For this review, take the finished solid that the model builds, in its own axes (mm). A direction names the side the tool comes from. Give positions to 0.01 mm unless a question says otherwise; leave off trailing zeros. Loops run counter-clockwise (first coordinate to the right, second up) from the corner with the lowest first, then second, coordinate; pieces in that order, holes last. Notation, with made-up numbers: (14.5, -0.5) -> (34.5, -0.5) arc R11 ccw to (34.5, 18.5) -> close; hole circle Ø3 at (88, 36.25). An arc over 180 degrees is marked (long way). Write each question's results on one line, items separated by ' | '. Start each with the question number.
```python
from build123d import *

# Parameters (mm, degrees)
SKETCH1_W                     = 190.5
SKETCH1_H                     = 101.6
BOSS_EXTRUDE1_DEPTH           = 1.5875
CONVERT_SOLID1_START          = -95.25
CONVERT_SOLID1_OUTLINE_W      = 3.175
CONVERT_SOLID1_OUTLINE_H      = 101.6
CONVERT_SOLID1_DEPTH          = 190.5
SKETCH30_R                    = 12.770921212
CUT_EXTRUDE6_DEPTH            = 38.1
SKETCH35_W                    = 139.601875342
SKETCH35_H                    = 6.35
CUT_EXTRUDE7_DEPTH            = 0.254
EDGE_FLANGE1_STRIP_W          = 39.05
EDGE_FLANGE1_STRIP_H          = 4.7625
EDGE_FLANGE1_STRIP_CUT_DEPTH  = 25.449062329
EDGE_FLANGE1_RELIEF_W         = 41.43125
EDGE_FLANGE1_RELIEF_H         = 2.38125
EDGE_FLANGE1_RELIEF_CUT_DEPTH = 4.7625
EDGE_FLANGE1_DEPTH            = 25.449062329
EDGE_FLANGE2_STRIP_W          = 39.05
EDGE_FLANGE2_STRIP_H          = 4.7625
EDGE_FLANGE2_STRIP_CUT_DEPTH  = 25.449062329
EDGE_FLANGE2_RELIEF_W         = 41.43125
EDGE_FLANGE2_RELIEF_H         = 2.38125
EDGE_FLANGE2_RELIEF_CUT_DEPTH = 4.7625
EDGE_FLANGE2_DEPTH            = 25.449062329
SKETCH45_W                    = 4.7625
SKETCH45_H                    = 0.000254
CUT_EXTRUDE10_DEPTH           = 25.4
EDGE_FLANGE4_STRIP_W          = 39.05
EDGE_FLANGE4_STRIP_H          = 4.7625
EDGE_FLANGE4_STRIP_CUT_DEPTH  = 25.4
EDGE_FLANGE4_RELIEF_W         = 41.43125
EDGE_FLANGE4_RELIEF_H         = 2.38125
EDGE_FLANGE4_RELIEF_CUT_DEPTH = 4.7625
EDGE_FLANGE4_DEPTH            = 25.4
FILLET9_R                     = 25.4
CUT_EXTRUDE11_DEPTH           = 25.4
FILLET10_R                    = 25.4
SKETCH53_R                    = 2.54
CUT_EXTRUDE12_DEPTH           = 4.7625
SKETCH54_R                    = 2.54
CUT_EXTRUDE13_DEPTH           = 4.7625
SKETCH55_R                    = 9.525
SKETCH55_R_2                  = 2.54
CUT_EXTRUDE14_DEPTH           = 4.7625


# Read off the part's stored shape, not the designer's step: Convert-Solid1
# Sheet-metal steps are written as plain solids
with BuildPart() as part:
    # Sketch1 → Boss-Extrude1 (new body)
    with BuildSketch(Plane(origin=(0, 0, 0), x_dir=(1, 0, 0), z_dir=(0, 1, 0))):
        Rectangle(SKETCH1_W, SKETCH1_H)
    extrude(amount=BOSS_EXTRUDE1_DEPTH)

    # Convert-Solid1 outline → Convert-Solid1 (add)
    with BuildSketch(Plane.YZ.offset(CONVERT_SOLID1_START)):
        with Locations((-1.5875, 0)):
            Rectangle(CONVERT_SOLID1_OUTLINE_W, CONVERT_SOLID1_OUTLINE_H)
    extrude(amount=CONVERT_SOLID1_DEPTH)

    # Sketch30 → Cut-Extrude6 (cut)
    with BuildSketch(Plane(origin=(0, -3.175, 0), x_dir=(-1, 0, 0), z_dir=(0, -1, 0))):
        with Locations(Location((0, -25.504506424, 0), (0, 0, 90))):
            Circle(SKETCH30_R)
    extrude(amount=-CUT_EXTRUDE6_DEPTH, mode=Mode.SUBTRACT)

    # Sketch35 → Cut-Extrude7 (cut)
    with BuildSketch(Plane(origin=(0, 0, -50.8), x_dir=(-1, 0, 0), z_dir=(0, 0, -1))):
        Rectangle(SKETCH35_W, SKETCH35_H)
    extrude(amount=-CUT_EXTRUDE7_DEPTH, mode=Mode.SUBTRACT)

    # Edge-Flange1 strip (across the edge) → Edge-Flange1 strip cut (cut)
    with BuildSketch(Plane(origin=(95.25, 1.5875, -50.8), x_dir=(0, 0, 1), z_dir=(-1, 0, 0))):
        with Locations((-4.7625, -2.38125)):
            Rectangle(EDGE_FLANGE1_STRIP_W, EDGE_FLANGE1_STRIP_H)
    extrude(amount=EDGE_FLANGE1_STRIP_CUT_DEPTH, mode=Mode.SUBTRACT)

    # Edge-Flange1 relief (on the sheet) → Edge-Flange1 relief cut (cut)
    with BuildSketch(Plane(origin=(95.25, 1.5875, -36.0375), x_dir=(0, 0, 1), z_dir=(0, 1, 0))):
        with Locations((-18.334375, -26.639687329)):
            Rectangle(EDGE_FLANGE1_RELIEF_W, EDGE_FLANGE1_RELIEF_H)
    extrude(amount=-EDGE_FLANGE1_RELIEF_CUT_DEPTH, mode=Mode.SUBTRACT)

    # Edge-Flange1 section (across the edge) → Edge-Flange1 (add)
    with BuildSketch(Plane(origin=(95.25, 1.5875, -50.8), x_dir=(0, 0, 1), z_dir=(-1, 0, 0))):
        with BuildLine():
            Line((0, 10), (0, 46.0375))
            Line((0, 46.0375), (4.7625, 46.0375))
            Line((4.7625, 46.0375), (4.7625, 10))
            ThreePointArc((4.7625, 10), (7.691432188, 2.928932188), (14.7625, 0))
            Line((14.7625, 0), (14.7625, -4.7625))
            ThreePointArc((14.7625, -4.7625), (4.323836143, -0.438663857), (0, 10))
        make_face()
    extrude(amount=EDGE_FLANGE1_DEPTH)

    # Edge-Flange2 strip (across the edge) → Edge-Flange2 strip cut (cut)
    with BuildSketch(Plane(origin=(-69.800937671, 1.5875, -50.8), x_dir=(0, 0, 1), z_dir=(-1, 0, 0))):
        with Locations((-4.7625, -2.38125)):
            Rectangle(EDGE_FLANGE2_STRIP_W, EDGE_FLANGE2_STRIP_H)
    extrude(amount=EDGE_FLANGE2_STRIP_CUT_DEPTH, mode=Mode.SUBTRACT)

    # Edge-Flange2 relief (on the sheet) → Edge-Flange2 relief cut (cut)
    with BuildSketch(Plane(origin=(-69.800937671, 1.5875, -36.0375), x_dir=(0, 0, 1), z_dir=(0, 1, 0))):
        with Locations((-18.334375, 1.190625)):
            Rectangle(EDGE_FLANGE2_RELIEF_W, EDGE_FLANGE2_RELIEF_H)
    extrude(amount=-EDGE_FLANGE2_RELIEF_CUT_DEPTH, mode=Mode.SUBTRACT)

    # Edge-Flange2 section (across the edge) → Edge-Flange2 (add)
    with BuildSketch(Plane(origin=(-69.800937671, 1.5875, -50.8), x_dir=(0, 0, 1), z_dir=(-1, 0, 0))):
        with BuildLine():
            Line((0, 10), (0, 46.0375))
            Line((0, 46.0375), (4.7625, 46.0375))
            Line((4.7625, 46.0375), (4.7625, 10))
            ThreePointArc((4.7625, 10), (7.691432188, 2.928932188), (14.7625, 0))
            Line((14.7625, 0), (14.7625, -4.7625))
            ThreePointArc((14.7625, -4.7625), (4.323836143, -0.438663857), (0, 10))
        make_face()
    extrude(amount=EDGE_FLANGE2_DEPTH)

    # Sketch45 → Cut-Extrude10 (cut)
    with BuildSketch(Plane(origin=(0, 1.5875, 0), x_dir=(1, 0, 0), z_dir=(0, 1, 0))):
        with Locations((-92.86875, -25.399873)):
            Rectangle(SKETCH45_W, SKETCH45_H)
        with Locations((-92.86875, 0.000381)):
            Rectangle(SKETCH45_W, SKETCH45_H)
    extrude(amount=-CUT_EXTRUDE10_DEPTH, mode=Mode.SUBTRACT)

    # Edge-Flange4 strip (across the edge) → Edge-Flange4 strip cut (cut)
    with BuildSketch(Plane(origin=(-95.25, 1.5875, -0.000254), x_dir=(1, 0, 0), z_dir=(0, 0, 1))):
        with Locations((-4.7625, -2.38125)):
            Rectangle(EDGE_FLANGE4_STRIP_W, EDGE_FLANGE4_STRIP_H)
    extrude(amount=EDGE_FLANGE4_STRIP_CUT_DEPTH, mode=Mode.SUBTRACT)

    # Edge-Flange4 relief (on the sheet) → Edge-Flange4 relief cut (cut)
    with BuildSketch(Plane(origin=(-80.4875, 1.5875, -0.000254), x_dir=(1, 0, 0), z_dir=(0, 1, 0))):
        with Locations((-18.334375, 1.190625)):
            Rectangle(EDGE_FLANGE4_RELIEF_W, EDGE_FLANGE4_RELIEF_H)
        with Locations((-18.334375, -26.590625)):
            Rectangle(EDGE_FLANGE4_RELIEF_W, EDGE_FLANGE4_RELIEF_H)
    extrude(amount=-EDGE_FLANGE4_RELIEF_CUT_DEPTH, mode=Mode.SUBTRACT)

    # Edge-Flange4 section (across the edge) → Edge-Flange4 (add)
    with BuildSketch(Plane(origin=(-95.25, 1.5875, -0.000254), x_dir=(1, 0, 0), z_dir=(0, 0, 1))):
        with BuildLine():
            Line((0, 10), (0, 20.6375))
            Line((0, 20.6375), (4.7625, 20.6375))
            Line((4.7625, 20.6375), (4.7625, 10))
            ThreePointArc((4.7625, 10), (7.691432188, 2.928932188), (14.7625, 0))
            Line((14.7625, 0), (14.7625, -4.7625))
            ThreePointArc((14.7625, -4.7625), (4.323836143, -0.438663857), (0, 10))
        make_face()
    extrude(amount=EDGE_FLANGE4_DEPTH)

    # Fillet9
    # the kernel refuses this fillet: 25.4 mm, written as the material it takes off along each edge
    with BuildSketch(Plane(origin=(-67.419687671, 61.417239936, -50.546), x_dir=(1, 0, 0), z_dir=(0, -1, 0))) as fillet9_piece_1:
        with BuildLine():
            CenterArc((23.931895975, 25.4), FILLET9_R, 199.575530564, 70.424469436)
            Line((0, 16.88975), (-0.478637919, 16.719545))
            ThreePointArc((-0.478637919, 16.719545), (-0.508, 8.444875), (-0.508, 0))
            Line((-0.508, 0), (0, -0.508))
            Line((0, -0.508), (23.931895975, -0.508))
            Line((23.931895975, -0.508), (23.931895975, 0))
        make_face()
    extrude(amount=124.421979873, mode=Mode.SUBTRACT)
    with BuildSketch(Plane(origin=(67.419687671, 61.417239936, -50.546), x_dir=(0, 0, 1), z_dir=(0, -1, 0))) as fillet9_piece_2:
        with BuildLine():
            CenterArc((25.4, 23.931895975), FILLET9_R, 180, 70.424469436)
            Line((0, 23.931895975), (-0.508, 23.931895975))
            Line((-0.508, 23.931895975), (-0.508, 0))
            Line((-0.508, 0), (0, -0.508))
            ThreePointArc((0, -0.508), (8.444875, -0.508), (16.719545, -0.478637919))
            Line((16.719545, -0.478637919), (16.88975, 0))
        make_face()
    extrude(amount=124.421979873, mode=Mode.SUBTRACT)

    # Sketch52 → Cut-Extrude11 (cut)
    with BuildSketch(Plane.XZ.offset(3.175)):
        with BuildLine():
            ThreePointArc((62.156767956, 50.8), (84.936935051, 40.486935051), (95.25, 17.706767956))
            Line((95.25, 17.706767956), (95.25, 50.8))
            Line((95.25, 50.8), (62.156767956, 50.8))
        make_face()
    extrude(amount=-CUT_EXTRUDE11_DEPTH, mode=Mode.SUBTRACT)

    # Fillet10
    # the kernel refuses this fillet: 25.4 mm, written as the material it takes off along each edge
    with BuildSketch(Plane(origin=(-95.25, 64.807891195, 50.8), x_dir=(1, 0, 0), z_dir=(0, -1, 0))) as fillet10_piece_1:
        with BuildLine():
            CenterArc((25.288156478, -25.4), FILLET10_R, 90, 84.621196501)
            Line((0, -23.019004), (-0.50576313, -22.97138408))
            ThreePointArc((-0.50576313, -22.97138408), (-0.508, -11.509502), (-0.508, 0))
            Line((-0.508, 0), (0, 0.508))
            Line((0, 0.508), (25.288156478, 0.508))
            Line((25.288156478, 0.508), (25.288156478, 0))
        make_face()
    extrude(amount=131.203282389, mode=Mode.SUBTRACT)

    # Sketch53 → Cut-Extrude12 (cut)
    with BuildSketch(Plane.ZY.offset(95.25)):
        with Locations(Location((6.349746, 17.9375, 0), (0, 0, 270))):
            Circle(SKETCH53_R)
        with Locations(Location((19.049746, 17.9375, 0), (0, 0, 270))):
            Circle(SKETCH53_R)
    extrude(amount=-CUT_EXTRUDE12_DEPTH, mode=Mode.SUBTRACT)

    # Sketch54 → Cut-Extrude13 (cut)
    with BuildSketch(Plane(origin=(0, 0, -50.8), x_dir=(-1, 0, 0), z_dir=(0, 0, -1))):
        with Locations(Location((-82.55, 34.925, 0), (0, 0, 90))):
            Circle(SKETCH54_R)
        with Locations(Location((82.55, 34.925, 0), (0, 0, 90))):
            Circle(SKETCH54_R)
    extrude(amount=-CUT_EXTRUDE13_DEPTH, mode=Mode.SUBTRACT)

    # Sketch55 → Cut-Extrude14 (cut)
    with BuildSketch(Plane.XZ.offset(3.175)):
        with Locations(Location((-39.37, -22.688605117, 0), (0, 0, 270))):
            Circle(SKETCH55_R)
        with Locations(Location((39.37, -22.688605117, 0), (0, 0, 270))):
            Circle(SKETCH55_R)
        with Locations(Location((-17.001810213, -34.722893033, 0), (0, 0, 270))):
            Circle(SKETCH55_R_2)
        with Locations(Location((-61.002047674, -9.376410953, 0), (0, 0, 270))):
            Circle(SKETCH55_R_2)
        with Locations(Location((61.002047674, -9.376410953, 0), (0, 0, 270))):
            Circle(SKETCH55_R_2)
        with Locations(Location((17.001810213, -34.722893033, 0), (0, 0, 270))):
            Circle(SKETCH55_R_2)
    extrude(amount=-CUT_EXTRUDE14_DEPTH, mode=Mode.SUBTRACT)


solid = part.part
```
1. We need section D-D (y = 5). Write out the cut boundary in (x, z), plus the area to 3 significant figures.
2. Wall thickness on L1, parallel to Z at x = -39, y = -1; L2, parallel to Y at x = 27, z = 32 (1 decimal); L3, parallel to Z at x = -70, y = 45.5: over which ranges is each line inside the solid? List them lowest first.
3. Machinability: for faces 5 (the flat face through (-93, 22.225, 13)), 6 (the flat face through (-87, -1, 27.781)), 7 (the cylindrical face through (-82.347, 4.595, -43.186)), 8 (the cylindrical face through (57.955, -0.76, -46.024)), 9 (the cylindrical face through (82.704, 1.035, -46.361)), which of the approach directions +Z, -Z, +X, -X, +Y, -Y give a long, thin tool a straight path to every point of the face, cutting with its end or side? Answer none if there is none.
4. We need section A-A (x = 39.37). Write out the cut boundary in (y, z) (1 decimal), plus the area to 3 significant figures.
5. For pin 1 Ø20.5 at (x, z) = (0, 25.5) entering from +Y; pin 2 Ø3 at (y, z) = (17, 14) entering from +X; pin 3 Ø2.5 at (y, z) = (-1, 26) entering from -X (3 decimals); pin 4 Ø25 at (x, z) = (39.37, -22.69) entering from -Y (3 decimals), all flat-tipped, find the tip position at first contact; note any pin that passes through.
6. We need section B-B (y = 27.5). Write out the cut boundary in (x, z), plus the area to 3 significant figures.
7. We need section C-C (z = -42). Count the separate pieces of the cut face and the enclosed holes in it, plus the area to 3 significant figures.
8. Draft analysis for pull direction Z (two halves, no side actions). For faces 1 (the cylindrical face through (-4.891, -0.827, 13.707)), 2 (the cylindrical face through (-86.865, -0.76, 44.359)), 3 (the flat face through (83, 47.625, -48)), 4 (the cylindrical face through (-58.312, -0.76, -45.772)), state which applies: released by +Z, released by -Z, zero draft, split by the parting line, or undercut.
Response:
1) outline: (-95.25, -49.25) -> (-69.8, -49.25) -> (-69.8, -43.56) -> (-95.25, -43.56) -> close; (-93.7, 0) -> (-88.01, 0) -> (-88.01, 25.4) -> (-93.7, 25.4) -> close; (69.8, -49.25) -> (95.25, -49.25) -> (95.25, -43.56) -> (69.8, -43.56) -> close | area: 434 mm2
2) L1: z = -50.55 to -32.21, -13.17 to 50.8 | L2: y = -3.2 to 1.6 | L3: z = -50.8 to -46.04
3) face 5: +Z, +X, -X, +Y | face 6: -X, +Y, -Y | face 7: +X, -X, +Y | face 8: -Z, +Y, -Y | face 9: -Z, +X, -Y
4) outline: (-3.2, -50.5) -> (1.6, -50.5) -> (1.6, -32.2) -> (-3.2, -32.2) -> close; (-3.2, -13.2) -> (1.6, -13.2) -> (1.6, 50.8) -> (-3.2, 50.8) -> close | area: 392 mm2
5) pin 1: passes through | pin 2: stops at x = -90.49 | pin 3: stops at x = -89.755 | pin 4: stops at y = -3.175
6) outline: (-95.25, -50.8) -> (-69.8, -50.8) -> (-69.8, -46.04) -> (-95.25, -46.04) -> close; (69.8, -50.8) -> (95.25, -50.8) -> (95.25, -46.04) -> (69.8, -46.04) -> close | area: 242 mm2
7) separate pieces: 3 | enclosed holes: 0 | area: 874 mm2
8) face 1: undercut | face 2: released by +Z | face 3: zero draft | face 4: released by -Z
